from build123d import *

# Parameters (mm, degrees)
EXTRUDE_1_DEPTH = 20
SKETCH_2_W      = 5
SKETCH_2_H      = 5
EXTRUDE_2_DEPTH = 25
FILLET_1_R      = 1


with BuildPart() as part:
    # 草图1 → 凸台-拉伸1 (new body)
    with BuildSketch(Plane.XY):
        Polygon((-10, 5), (-10, 12), (-3.333333333, 5), (-3.333333333, 12), (3.333333333, 5), (3.333333333, 12), (10, 5), (10, -5), (-10, -5), align=None)
    extrude(amount=EXTRUDE_1_DEPTH)

    # 草图2 → 凸台-拉伸2 (add)
    with BuildSketch(Plane.XZ.offset(5)):
        with Locations((-7.5, 17.5)):
            Rectangle(SKETCH_2_W, SKETCH_2_H)
    extrude(amount=-EXTRUDE_2_DEPTH)

    # 圆角1
    fillet_1_edges = [part.edges().sort_by_distance(p)[0] for p in [
        (-10, 7.5, 20),
        (10, 0, 20),
        (-7.5, 20, 20),
        (-7.5, 20, 15),
        (-10, 20, 17.5),
        (-5, 20, 17.5),
        (10, 0, 0),
        (-10, 3.5, 0),
    ]]
    fillet(fillet_1_edges, radius=FILLET_1_R)


solid = part.part
Verification items for the finished model (mm, model axes). A direction names the side the tool comes from. Round coordinates to 2 decimals unless told otherwise and drop trailing zeros. Loops run counter-clockwise (first coordinate to the right, second up) from the corner with the lowest first, then second, coordinate; pieces in that order, holes last. Notation, with made-up numbers: M 1,29.5 L 26,29.5 A18 ccw 26,58.5 Z; hole C -18.75,9.25 d9. An arc over 180 degrees is marked long. Write each question's results on one line, items separated by ' | '.
1) Section check C-C on x = 8. Record the boundary of the cut face in (y, z), then the cut area to 3 significant figures.
Checks:
outline: M -5,0 L 7.1,0 L 7.1,20 L -5,20 Z | area: 242 mm2
2) Section check A-A on z = 17.75. Record the boundary of the cut face in (x, y), then the cut area to 3 significant figures.
Checks:
outline: M -10,-5 L 10,-5 L 10,5 L 3.33,12 L 3.33,5 L -3.33,12 L -3.33,5 L -5,6.75 L -5,19 A1 ccw -6,20 L -9,20 A1 ccw -10,19 Z | area: 323 mm2
3) Scan lines: L1, parallel to Z at x = -7.25, y = 11.25; L2, parallel to X at y = 9.5, z = 12; L3, parallel to X at y = 10, z = 4.5. Record each from-to range of solid material in increasing order. Write a range as from..to.
Checks:
L1: z = 15..20 | L2: x = -10..-7.62, -3.33..-0.95, 3.33..5.71 | L3: x = -10..-8.1, -3.33..-1.43, 3.33..5.24
4) Section check D-D on z = 8.5. Record the boundary of the cut face in (x, y).
Checks:
outline: M -10,-5 L 10,-5 L 10,5 L 3.33,12 L 3.33,5 L -3.33,12 L -3.33,5 L -10,12 Z
5) Access from +Z, -Z, +X, -X, +Y, -Y to the whole of each face (thin tool, end or side, straight path). Record for faces 1 (the flat face through (-3.333, 8, 10)), 2 (the flat face through (-8, 20, 18)), 3 (the flat face through (-6.713, 8.549, 7.638)).
Checks:
face 1: +Z, -Z, +Y | face 2: +Z, -Z, +X, -X, +Y | face 3: -Z, +Y
6) Mould release check, pull along X, two halves, no side actions. Record for faces 4 (the cylindrical face through (9.699, 0.448, 19.715)), 5 (the flat face through (-10, 5, 10)), 6 (the flat face through (-5, 13, 17)): released by +X, released by -X, zero draft, split by the parting line, or undercut.
Checks:
face 4: released by +X | face 5: released by -X | face 6: undercut
7) Gauge pin test, flat ends, axial feed: P1, Ø1.5, axis at y = 8, z = 3.5, coming from the +X side; P2, Ø1, axis at x = -3.5, z = 11, coming from the +Y side; P3, Ø5, axis at y = 9, z = 15, coming from the +X side. Record the tip position at first contact, or that the pin passes through.
Checks:
P1: stops at x = 7.86 | P2: stops at y = 12 | P3: stops at x = 8.57
8) Section check B-B on y = 18. Record the boundary of the cut face in (x, z), then the cut area to 3 significant figures.
Checks:
outline: M -10,15 L -5,15 L -5,20 L -9,20 A1 ccw -10,19 Z | area: 24.8 mm2
